from build123d import *

# Parameters (mm, degrees)
F0_W     = 81.28
F0_H     = 171.45
F1_DEPTH = 6.35
F2_W     = 57.15
F2_H     = 69.85
F3_DEPTH = 25.4
F4_W     = 40.64
F4_H     = 22.86
F5_DEPTH = 12.7
F6_W     = 4.938572
F6_H     = 47.53778
F6_W_2   = 2.998928
F7_DEPTH = 15.875


with BuildPart() as f1:
    # F0 (on Top) → F1 (new body)
    with BuildSketch(Plane.XY):
        with Locations((-47.749023, 24.367116)):
            Rectangle(F0_W, F0_H)
    extrude(amount=F1_DEPTH)

    # F2 (on face) → F3 (join)
    with BuildSketch(Plane.XY.offset(6.35)):
        with Locations((-49.99557, 44.730341)):
            Rectangle(F2_W, F2_H)
    extrude(amount=F3_DEPTH)

    # F4 (on face) → F5 (join)
    with BuildSketch(Plane.XY.offset(6.35)):
        with Locations((-49.00288, 95.77399)):
            Rectangle(F4_W, F4_H)
    extrude(amount=F5_DEPTH)

    # F6 (on face) → F7 (join)
    with BuildSketch(Plane.XY.offset(6.35)):
        Polygon((-49.00288, -13.820104), (-52.001808, -13.820104), (-52.001808, -91.607604), (-44.064308, -91.607604), (-44.064308, -13.820104), align=None)
        with Locations((-46.533594, -37.588994)):
            Rectangle(F6_W, F6_H)
        with Locations((-50.502344, -37.588994)):
            Rectangle(F6_W_2, F6_H)
    extrude(amount=F7_DEPTH)


solid = f1.part
Can you work these out from the model? Positions are in its coordinate system, mm. A direction names the side the tool comes from. Give positions to 0.01 mm unless a question says otherwise; leave off trailing zeros. Order: outer loops, then holes, each group sorted by start corner. A loop starts at its lowest first (then second) coordinate and runs counter-clockwise, first axis right, second up. Notation, with made-up numbers: M 78.25,18 L 93.25,18 A23 cw 93.25,49 Z; hole C -10.75,59 d1. An arc over 180 degrees is marked long. One line per item, written item: value.
Item 1: If we section it at C-C on x = -62.5: Write out the boundary of the cut face in (y, z), and give its area (3 significant figures).
Verdict:
outline: M -61.36,0 L 110.09,0 L 110.09,6.35 L 107.2,6.35 L 107.2,19.05 L 84.34,19.05 L 84.34,6.35 L 79.66,6.35 L 79.66,31.75 L 9.81,31.75 L 9.81,6.35 L -61.36,6.35 Z
area: 3,150 mm2
Item 2: If we mould it in two halves opening along Y, with no side actions, what happens to faces 1 (the face through (-50, 79.655, 19)), 2 (the face through (-7.109, 23, 3)), 3 (the face through (-48, -61.358, 3))? For each: pulls with the +Y half, pulls with the -Y half, needs draft (parallel to the pull), parting line crosses it, or undercut.
Verdict:
face 1: undercut
face 2: needs draft
face 3: pulls with the -Y half
Item 3: If we section it at A-A on z = 9.5: Write out the boundary of the cut face in (x, y), and give its area (3 significant figures).
Verdict:
outline: M -78.57,9.81 L -21.42,9.81 L -21.42,79.66 L -78.57,79.66 Z; M -69.32,84.34 L -28.68,84.34 L -28.68,107.2 L -69.32,107.2 Z; M -52,-91.61 L -44.06,-91.61 L -44.06,-13.82 L -52,-13.82 Z
area: 5,540 mm2
Item 4: For pin 1 (11.5 mm diameter, centred on x = -55.5, y = 91.5, fed in from +Z); pin 2 (6.5 mm diameter, centred on x = -46, y = -59, fed in from +Z) (3 decimals); pin 3 (4 mm diameter, centred on x = -55, z = 13.5, fed in from +Y), each with a flat end and sliding along its axis, tell me the tip position at first contact or that it passes through.
Verdict:
pin 1: z = 19.05
pin 2: z = 22.225
pin 3: y = 107.2
Item 5: Please list where these lines run through material, in increasing order: line 1 (Y direction, x = -44.5, z = 15); line 2 (Y direction, x = -29, z = 14.5); line 3 (Z direction, x = -13.5, y = -59).
Verdict:
line 1: -91.61 to -13.82, 9.81 to 79.66, 84.34 to 107.2
line 2: 9.81 to 79.66, 84.34 to 107.2
line 3: 0 to 6.35
Item 6: For faces 4 (the face through (-52.002, -52, 14)), 5 (the face through (-78.571, 44, 19)), 6 (the face through (-49, 96, 19.05)), 7 (the face through (-49, 84.344, 13)), 8 (the face through (-69.323, 96, 13)), which set-ups out of +Z, -Z, +X, -X, +Y, -Y let a thin tool reach every point of the face, with its end or its side?
Verdict:
face 4: +Z, -X, -Y
face 5: +Z, -X, +Y, -Y
face 6: +Z, +X, -X, +Y
face 7: +Z, +X, -X
face 8: +Z, -X, +Y
Item 7: If we section it at D-D on z = 29.5: Write out the boundary of the cut face in (x, y), and give its area (3 significant figures).
Verdict:
outline: M -78.57,9.81 L -21.42,9.81 L -21.42,79.66 L -78.57,79.66 Z
area: 3,990 mm2
Item 8: If we section it at B-B on y = 27: Write out the boundary of the cut face in (x, z).
Verdict:
outline: M -88.39,0 L -7.11,0 L -7.11,6.35 L -21.42,6.35 L -21.42,31.75 L -78.57,31.75 L -78.57,6.35 L -88.39,6.35 Z
